from build123d import *

# Parameters (mm, degrees)
F1_DEPTH  = 50.8
F3_DEPTH  = 76.201
F4_R      = 11.1125
F1_FACE_W = 76.2
F1_FACE_H = 50.8
F5_DEPTH  = 76.201
F6_R      = 5.08


with BuildPart() as f1:
    # F0 (on Front) → F1 (new body)
    with BuildSketch(Plane.XZ):
        Polygon((0, 76.2), (0, 0), (6.35, 0), (6.35, 69.85), (76.2, 69.85), (76.2, 76.2), align=None)
    extrude(amount=F1_DEPTH)

    # F2 (on Right) → F3 (cut, through all)
    with BuildSketch(Plane.YZ):
        with BuildLine():
            Line((-33.3375, 31.75), (-33.3375, 27.78125))
            ThreePointArc((-33.3375, 27.78125), (-25.4, 19.84375), (-17.4625, 27.78125))
            Line((-17.4625, 27.78125), (-17.4625, 31.75))
            Line((-17.4625, 31.75), (-33.3375, 31.75))
        make_face()
        with BuildLine():
            Line((-33.3375, 35.71875), (-33.3375, 31.75))
            Line((-33.3375, 31.75), (-17.4625, 31.75))
            Line((-17.4625, 31.75), (-17.4625, 35.71875))
            ThreePointArc((-17.4625, 35.71875), (-25.4, 43.65625), (-33.3375, 35.71875))
        make_face()
    extrude(amount=F3_DEPTH, mode=Mode.SUBTRACT)

    # F4 (on Top) + F1_face (on face) → F5 (cut, through all)
    with BuildSketch(Plane.XY):
        with Locations((38.1, -25.4)):
            Circle(F4_R)
    with BuildSketch(Plane(origin=(38.1, -25.4, 76.2), x_dir=(1, 0, 0), z_dir=(0, 0, 1))):
        Rectangle(F1_FACE_W, F1_FACE_H)
    extrude(amount=F5_DEPTH, mode=Mode.SUBTRACT)

    # F6
    f6_edges = [f1.edges().sort_by_distance(p)[0] for p in [
        (6.35, -25.4, 69.85),
        (76.2, -25.4, 69.85),
        (6.35, -25.4, 0),
    ]]
    fillet(f6_edges, radius=F6_R)


solid = f1.part
Model file for the job. Use its own axes, mm. A direction names the side the tool comes from. Give positions to 0.01 mm unless a question says otherwise; leave off trailing zeros. Order: outer loops, then holes, each group sorted by start corner. A loop starts at its lowest first (then second) coordinate and runs counter-clockwise, first axis right, second up. Notation, with made-up numbers: (4.25, -25.75) - (40.25, -25.75) arc R26 cw to (40.25, 13.25) - close; hole circle Ø3 at (-6.5, 55). An arc over 180 degrees is marked (long way). One line per item, written item: value.
Item 1: Two-plate mould, pull along Y, no slides. Class faces 4 (the flat face through (3, -33.338, 32)), 5 (the cylindrical face through (74.751, -25.756, 71.378)), 6 (the flat face through (4, -50.8, 55)): released by +Y, released by -Y, zero draft, split by the parting line, or undercut.
Response values:
face 4: undercut
face 5: zero draft
face 6: released by -Y
Item 2: Slice it at B-B (y = -20). List the corners of the cut face in (x, z).
Response values:
outline: (0, 0) - (1.27, 0) arc R5.08 ccw to (6.35, 5.08) - (6.35, 21.96) - (0, 21.96) - close; (0, 41.54) - (6.35, 41.54) - (6.35, 64.77) arc R5.08 cw to (11.43, 69.85) - (28.39, 69.85) - (28.39, 76.2) - (0, 76.2) - close; (47.81, 69.85) - (71.12, 69.85) arc R5.08 ccw to (76.2, 74.93) - (76.2, 76.2) - (47.81, 76.2) - close
Item 3: Slice it at D-D (x = 57). List the corners of the cut face in (y, z).
Response values:
outline: (-50.8, 69.85) - (0, 69.85) - (0, 76.2) - (-50.8, 76.2) - close
Item 4: Tool access for faces 1 (the cylindrical face through (48.7, -22.06, 72.98)), 2 (the flat face through (6.35, -19, 41)), 3 (the cylindrical face through (3.131, -25.575, 19.846)): list every direction of +Z, -Z, +X, -X, +Y, -Y with a clear straight run to the whole face (end or side of a thin tool).
Response values:
face 1: +Z, -Z
face 2: -Z, +X, +Y, -Y
face 3: +X, -X
Item 5: Wall check: line 1 (Y direction, x = 38, z = 72); line 2 (X direction, y = -25.4, z = 74.5); line 3 (Z direction, x = 18, y = -35). Give the ranges that are in metal, low to high.
Response values:
line 1: -50.8 to -36.51, -14.29 to 0
line 2: 0 to 26.99, 49.21 to 76.18
line 3: 69.85 to 76.2
Item 6: Slice it at A-A (x = 38.1). List the corners of the cut face in (y, z).
Response values:
outline: (-50.8, 69.85) - (-36.51, 69.85) - (-36.51, 76.2) - (-50.8, 76.2) - close; (-14.29, 69.85) - (0, 69.85) - (0, 76.2) - (-14.29, 76.2) - close
Item 7: Pin check, flat tips, straight feed: pin 1 Ø6 at (x, y) = (16, -19) entering from -Z; pin 2 Ø1.5 at (y, z) = (-11.5, 15) entering from +X; pin 3 Ø12 at (x, z) = (38.5, 58.5) entering from -Y; pin 4 Ø2 at (y, z) = (-23.5, 65.5) entering from +X. Stop position of each tip, or through.
Response values:
pin 1: z = 69.85
pin 2: x = 6.35
pin 3: through
pin 4: x = 6.65
Item 8: Slice it at C-C (y = -6.5). List the corners of the cut face in (x, z).
Response values:
outline: (0, 0) - (1.27, 0) arc R5.08 ccw to (6.35, 5.08) - (6.35, 64.77) arc R5.08 cw to (11.43, 69.85) - (71.12, 69.85) arc R5.08 ccw to (76.2, 74.93) - (76.2, 76.2) - (0, 76.2) - close
